```python
from build123d import *

# Parameters (mm, degrees)
F0_W     = 914.4
F0_H     = 25.4
F2_DEPTH = 457.2
F3_DEPTH = 457.2
F5_DEPTH = 304.8


with BuildPart() as f2:
    # F0 (on Front) → F2 (new body, symmetric)
    with BuildSketch(Plane.XZ):
        with Locations((0, 12.7)):
            Rectangle(F0_W, F0_H)
    extrude(amount=F2_DEPTH, both=True)

    # F1 (on Front) → F3 (join, symmetric)
    with BuildSketch(Plane.XZ):
        Polygon((0, 0), (-35.921024, 0), (-251.447171, -215.526147), (-251.447171, -251.447171), align=None)
        Polygon((35.921024, 0), (0, 0), (251.447171, -251.447171), (251.447171, -215.526147), align=None)
    extrude(amount=F3_DEPTH, both=True)

    # F4 (on Front) → F5 (cut, symmetric)
    with BuildSketch(Plane.XZ):
        Polygon((0, 0), (-35.921024, 0), (-251.447171, -215.526147), (-251.447171, -251.447171), align=None)
        Polygon((35.921024, 0), (0, 0), (251.447171, -251.447171), (251.447171, -215.526147), align=None)
    extrude(amount=F5_DEPTH, both=True, mode=Mode.SUBTRACT)


solid = f2.part
```
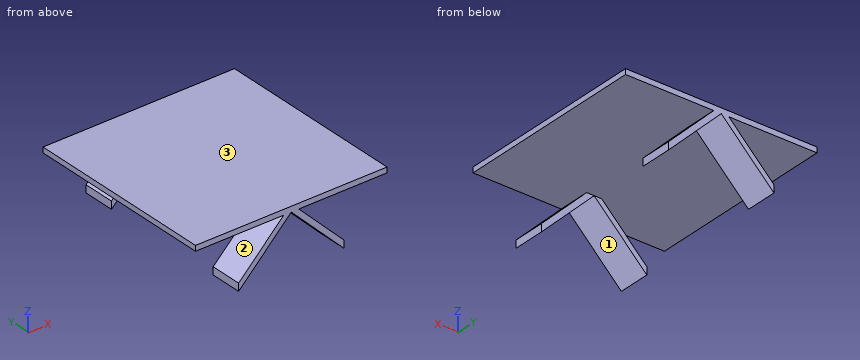
Can you work these out from the model? Positions are in its coordinate system, mm. Face numbers are marked on the shaded views. Coordinates: 2 decimals unless noted, no trailing zeros. Loops run counter-clockwise (first coordinate to the right, second up) from the corner with the lowest first, then second, coordinate; pieces in that order, holes last. Notation, with made-up numbers: (72.25, -0.75) -> (88.25, -0.75) arc R15 ccw to (88.25, 21.25) -> close; hole circle Ø5 at (15.5, 39.25). An arc over 180 degrees is marked (long way). Answer as a JSON object with one key per item and string values.
1) Imagine slicing it at B-B (z = -228). Please give me the cut outline in (x, y), then the cut area to 3 significant figures.
Results:
{"outline": "(-251.45, -457.2) -> (-228, -457.2) -> (-228, -304.8) -> (-251.45, -304.8) -> close; (-251.45, 304.8) -> (-228, 304.8) -> (-228, 457.2) -> (-251.45, 457.2) -> close; (228, -457.2) -> (251.45, -457.2) -> (251.45, -304.8) -> (228, -304.8) -> close; (228, 304.8) -> (251.45, 304.8) -> (251.45, 457.2) -> (228, 457.2) -> close", "area": "14,300 mm^2"}
2) Imagine slicing it at A-A (y = 337.5). Please give me the cut outline in (x, z), then the cut area to 3 significant figures.
Results:
{"outline": "(-457.2, 0) -> (-35.92, 0) -> (-251.45, -215.53) -> (-251.45, -251.45) -> (0, 0) -> (251.45, -251.45) -> (251.45, -215.53) -> (35.92, 0) -> (457.2, 0) -> (457.2, 25.4) -> (-457.2, 25.4) -> close", "area": "40,000 mm^2"}
3) Thinking about a two-plate mould opening in Z: for the marked faces 1, 2 and 3, which applies, pulls with the +Z half, pulls with the -Z half, needs draft (parallel to the pull), parting line crosses it, or undercut?
Results:
{"face 1": "pulls with the -Z half", "face 2": "undercut", "face 3": "pulls with the +Z half"}
4) Imagine slicing it at D-D (z = -67). Please give me the cut outline in (x, y).
Results:
{"outline": "(-102.92, -457.2) -> (-67, -457.2) -> (-67, -304.8) -> (-102.92, -304.8) -> close; (-102.92, 304.8) -> (-67, 304.8) -> (-67, 457.2) -> (-102.92, 457.2) -> close; (67, -457.2) -> (102.92, -457.2) -> (102.92, -304.8) -> (67, -304.8) -> close; (67, 304.8) -> (102.92, 304.8) -> (102.92, 457.2) -> (67, 457.2) -> close"}
5) If I drill on line 1 (Z direction, x = -299, y = -11); line 2 (X direction, y = -360, z = -205.5); line 3 (Z direction, x = -1.5, y = -353), over which ranges is the centre line in solid material (lowest first)?
Results:
{"line 1": "z = 0 to 25.4", "line 2": "x = -241.42 to -205.5, 205.5 to 241.42", "line 3": "z = -1.5 to 25.4"}
6) Imagine slicing it at C-C (x = -56.5). Please give me the cut outline in (y, z).
Results:
{"outline": "(-457.2, -56.5) -> (-304.8, -56.5) -> (-304.8, -20.58) -> (-457.2, -20.58) -> close; (-457.2, 0) -> (457.2, 0) -> (457.2, 25.4) -> (-457.2, 25.4) -> close; (304.8, -56.5) -> (457.2, -56.5) -> (457.2, -20.58) -> (304.8, -20.58) -> close"}
7) For P1, Ø1, axis at x = 170, y = -9, coming from the -Z side; P2, Ø4, axis at x = 182.5, y = 307, coming from the -Z side; P3, Ø18, axis at y = 353.5, z = -237, coming from the +X side, each with a flat end and sliding along its axis, tell me the tip position at first contact or that it passes through.
Results:
{"P1": "stops at z = 0", "P2": "stops at z = -184.5", "P3": "stops at x = 251.45"}
